Verification items for the finished model (mm, model axes). A direction names the side the tool comes from. Round coordinates to 2 decimals unless told otherwise and drop trailing zeros. Write each loop counter-clockwise with the first axis right and the second up, starting at its lowest first coordinate (ties: lowest second). Pieces come first, ordered by that corner, then holes. Notation, with made-up numbers: (26.25, 36.25) -> (32.25, 36.25) arc R14 cw to (32.25, 50.25) -> close; hole circle Ø8 at (37, -21.5). An arc over 180 degrees is marked (long way). Answer as a JSON object with one key per item and string values. Group by question number.
(1) Set-up check for faces 5 (the face through (4, 0, 37)), 6 (the face through (6, 0, 1)), 7 (the face through (-5.875, 0, 68)): record each of +Z, -Z, +X, -X, +Y, -Y from which the full face is reachable in a straight line by a thin tool's end or side.
(2) Scan lines: L1, parallel to Z at x = 6.75, y = 0; L2, parallel to X at y = -0.5, z = 7; L3, parallel to Z at x = 5.7, y = 0. Record each from-to range of solid material in increasing order. Write a range as from..to.
(3) Sectioned sample at A-A on y = 5.75. Record the cut outline in (x, z) (3 decimals), and give its area (3 significant figures).
(4) Sectioned sample at C-C on z = 23. Record the cut outline in (x, y).
(5) Sectioned sample at B-B on x = 1. Record the cut outline in (y, z) (3 decimals).
(6) Gauge pin test, flat ends, axial feed: pin 1 Ø1.3 at (x, z) = (1, 67.5) entering from -Y; pin 2 Ø1.3 at (y, z) = (-2, 67) entering from -X (3 decimals); pin 3 Ø2.5 at (y, z) = (0, 3) entering from +X. Record the tip position at first contact, or that the pin passes through.
(7) Draft check along Z on faces 1 (the face through (-5, 0, 5)), 2 (the face through (0, 7, 37)), 3 (the face through (6.76, -0.325, 1.536)), 4 (the face through (-5, 0, 70)). Enter one of: released by +Z, released by -Z, zero draft, split by the parting line, or undercut.
(8) Sectioned sample at D-D on y = 0. Count the separate pieces of the cut face and the enclosed holes in it, and give its area (3 significant figures).
```python
from build123d import *

# Parameters (mm, degrees)
F0_W     = 15
F0_H     = 20
F0_W_2   = 8
F0_H_2   = 14
F1_DEPTH = 70
F2_W     = 18.400512
F2_H     = 24.49468
F2_W_2   = 11.75
F2_H_2   = 16.5
F3_DEPTH = 4.5
F4_R     = 1.75
F4_R_2   = 1.5
F5_DEPTH = 25
F6_W     = 12
F6_H     = 16.75
F7_DEPTH = 5


with BuildPart() as f1:
    # F0 (on Top) → F1 (new body)
    with BuildSketch(Plane.XY):
        Rectangle(F0_W, F0_H)
        Rectangle(F0_W_2, F0_H_2, mode=Mode.SUBTRACT)
    extrude(amount=F1_DEPTH)

    # F2 (on face) → F3 (cut)
    with BuildSketch(Plane.XY.offset(70)):
        Rectangle(F2_W, F2_H)
        Rectangle(F2_W_2, F2_H_2, mode=Mode.SUBTRACT)
    extrude(amount=-F3_DEPTH, mode=Mode.SUBTRACT)

    # F4 (on face) → F5 (cut)
    with BuildSketch(Plane.YZ.offset(7.5)):
        with Locations((0, 59.5)):
            Circle(F4_R)
        with Locations((0, 3)):
            Circle(F4_R_2)
    extrude(amount=-F5_DEPTH, mode=Mode.SUBTRACT)

    # F6 (on face) → F7 (cut)
    with BuildSketch(Plane(origin=(0, 0, 0), x_dir=(1, 0, 0), z_dir=(0, 0, -1))):
        Rectangle(F6_W, F6_H)
    extrude(amount=-F7_DEPTH, mode=Mode.SUBTRACT)


solid = f1.part
```
Computed values:
{
 "1": {"face 5": "+Z, -Z", "face 6": "-Z", "face 7": "+Z, -X, +Y, -Y"},
 "2": {"L1": "0..1.5, 4.5..57.75, 61.25..65.5", "L2": "-7.5..-4, 4..7.5", "L3": "5..57.75, 61.25..70"},
 "3": {"outline": "(-7.5, 0) -> (-6, 0) -> (-6, 5) -> (-4, 5) -> (-4, 70) -> (-5.875, 70) -> (-5.875, 65.5) -> (-7.5, 65.5) -> close; (4, 5) -> (6, 5) -> (6, 0) -> (7.5, 0) -> (7.5, 65.5) -> (5.875, 65.5) -> (5.875, 70) -> (4, 70) -> close", "area": "455 mm2"},
 "4": {"outline": "(-7.5, -10) -> (7.5, -10) -> (7.5, 10) -> (-7.5, 10) -> close; hole (-4, -7) -> (4, -7) -> (4, 7) -> (-4, 7) -> close"},
 "5": {"outline": "(-10, 0) -> (-8.375, 0) -> (-8.375, 5) -> (-7, 5) -> (-7, 70) -> (-8.25, 70) -> (-8.25, 65.5) -> (-10, 65.5) -> close; (7, 5) -> (8.375, 5) -> (8.375, 0) -> (10, 0) -> (10, 65.5) -> (8.25, 65.5) -> (8.25, 70) -> (7, 70) -> close"},
 "6": {"pin 1": "y = -8.25", "pin 2": "x = -5.875", "pin 3": "through"},
 "7": {"face 1": "released by -Z", "face 2": "zero draft", "face 3": "undercut", "face 4": "released by +Z"},
 "8": {"separate pieces": "6", "enclosed holes": "0", "area": "422 mm2"}
}
